Autodesk Fusion 360 part; units mm, degrees
sketch "Sketch1" plane through (0, 0, 0) normal (0, 0, 1) x (1, 0, 0) in component "clamp"
  circle A0 centre (60, 60) radius 27
  circle A1 centre (240, 60) radius 27
  arc A2 (210.2752, 14.9174) -> (89.7248, 14.9174) centre (150, -76.5) ccw
  arc A3 (89.7248, 105.0826) -> (210.2752, 105.0826) centre (150, 196.5) ccw
  arc A4 (89.7248, 105.0826) -> (89.7248, 14.9174) centre (60, 60) ccw
  arc A5 (210.2752, 14.9174) -> (210.2752, 105.0826) centre (240, 60) ccw
  dimension "d1" = 54
  dimension "d2" = 54
  dimension "d6" = 180
  dimension "d9" = 54
  dimension "d10" = 54
extrude "Extrude1" add sketch "Sketch1" along normal blind 13 makes body 1 in component "clamp"
extrude "Extrude1'" add sketch "Sketch1" along normal blind 12.7 separate body makes body 2
component "clamp" placed x (1, 0, 0) y (0, 1, 0) z (0, 0, 1) at (0, 0, 0)
hidden bodies 1
equation "d2 = d1"
equation "d9 = d1"
equation "d10 = d1"
equation "d17 = 1/2\""
Build history of the part. All positions in model axes, mm. Round coordinates to 2 decimals unless told otherwise and drop trailing zeros. Write each loop counter-clockwise with the first axis right and the second up, starting at its lowest first coordinate (ties: lowest second). Pieces come first, ordered by that corner, then holes. Notation, with made-up numbers: M 39,36 L 91,36 A20 cw 91,58 Z; hole C -21,-23.5 d1. An arc over 180 degrees is marked long. Use CSV: the item, a comma, the result in double quotes.
1. Two-plate mould, pull along Y, no slides. Class faces 1 (the face through (150.894, 87.004, 6.261)), 2 (the face through (6.025, 58.372, 6.261)), 3 (the face through (85.753, 51.89, 6.261)): +Y half, -Y half, draft (parallel to the pull), parting line (faces both ways), or undercut.
Reply:
face 1,"+Y half"
face 2,"parting line"
face 3,"undercut"
2. Saw through at D-D (y = 26). Give the cut face in (x, z).
Reply:
outline,"M 18.05,0 L 111.48,0 L 111.48,12.7 L 18.05,12.7 Z; M 188.52,0 L 281.95,0 L 281.95,12.7 L 188.52,12.7 Z"
3. Saw through at B-B (y = 52). Give the cut face in (x, z), plus the area to 3 significant figures.
Reply:
outline,"M 6.6,0 L 34.21,0 L 34.21,12.7 L 6.6,12.7 Z; M 85.79,0 L 214.21,0 L 214.21,12.7 L 85.79,12.7 Z; M 265.79,0 L 293.4,0 L 293.4,12.7 L 265.79,12.7 Z"
area,"2,330 mm²"
4. Saw through at A-A (x = 60). Give the cut face in (y, z).
Reply:
outline,"M 6,0 L 33,0 L 33,12.7 L 6,12.7 Z; M 87,0 L 114,0 L 114,12.7 L 87,12.7 Z"
5. Saw through at C-C (z = 10.25). Give the cut face in (x, y), plus the area to 3 significant figures.
Reply:
outline,"M 89.72,14.92 A109.5 cw 210.28,14.92 A54 ccw long 210.28,105.08 A109.5 cw 89.72,105.08 A54 ccw long Z; hole C 60,60 d54; hole C 240,60 d54"
area,"18,600 mm²"
6. Wall check: probe 1 along Y at (x, z) = (240, 7.5); probe 2 along X at (y, z) = (78.5, 9.25); probe 3 along X at (y, z) = (103, 2.75). Give the ranges that are in metal, low to high. Write a range as from..to.
Reply:
probe 1,"y = 6..33, 87..114"
probe 2,"x = 9.27..40.33, 79.67..220.33, 259.67..290.73"
probe 3,"x = 27.33..93.01, 206.99..272.67"
7. Flat gauge pins, fed straight in: pin 1 (4 mm diameter, centred on y = 45, z = 4.5, fed in from -X); pin 2 (4 mm diameter, centred on x = 172.5, z = 7.5, fed in from +Y); pin 3 (6 mm diameter, centred on x = 82, z = 11, fed in from +Y). Where does each tip first touch, or does it go through?
Reply:
pin 1,"stops at x = 7.59"
pin 2,"stops at y = 89.78"
pin 3,"stops at y = 110.55"
